The model under review builds one solid part; all positions refer to its coordinate system, in mm. Face numbers are marked on the shaded views. A direction names the side the tool comes from. Coordinates: 2 decimals unless noted, no trailing zeros. Order: outer loops, then holes, each group sorted by start corner. A loop starts at its lowest first (then second) coordinate and runs counter-clockwise, first axis right, second up. Notation, with made-up numbers: (51, -30) -> (60, -30) arc R19 cw to (60, -23) -> close; hole circle Ø1 at (-15.5, 54.25). An arc over 180 degrees is marked (long way). Put each result on its own line as item: value.
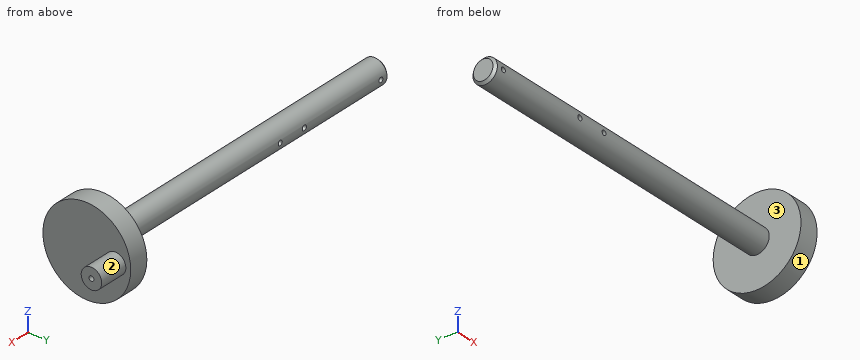
Autodesk Inventor part; units mm, degrees
ref_plane "YZ Plane" through (0, 0, 0) normal (1, 0, 0) x (0, 1, 0)
ref_plane "XZ Plane" through (0, 0, 0) normal (0, 1, 0) x (-1, 0, 0)
ref_plane "XY Plane" through (0, 0, 0) normal (0, 0, 1) x (1, 0, 0)
sketch "Sketch1" plane through (0, 0, 0) normal (0, 0, 1) x (1, 0, 0)
  line L0 (0, 0) -> (72, 0)
  line L1 (68, 2.5) -> (0, 2.5)
  line L2 (0, 2.5) -> (0, 0)
  line L3 (68, 2.5) -> (68, 9)
  line L4 (68, 9) -> (72, 9)
  line L5 (72, 9) -> (72, 0)
revolve "Revolution1" add sketch "Sketch1" angle 360 about axis through (0, 0, 0) along (1, 0, 0)
chamfer "Chamfer1" distance 0.5 angle 45 1 edges at (0, -2.5, 0)
thread "Thread1"
sketch "Sketch2" plane through (72, 0, 0) normal (1, 0, 0) x (0, 0, -1)
  circle A0 centre (0, 5.9) radius 2.1
  circle A1 centre (0, 5.9) radius 0.5
extrude "Extrusion1" add sketch "Sketch2" along normal blind 6
sketch "Sketch3" plane through (0, 0, 0) normal (0, 1, 0) x (-1, 0, 0)
  circle A0 centre (-2, 0) radius 0.5
extrude "Extrusion2" cut sketch "Sketch3" along normal mid plane 10
sketch "Sketch4" plane through (0, 0, 0) normal (0, 1, 0) x (-1, 0, 0)
  circle A0 centre (-27, 0) radius 0.5
extrude "Extrusion3" cut sketch "Sketch4" along normal mid plane 10
sketch "Sketch5" plane through (0, 0, 0) normal (0, 1, 0) x (-1, 0, 0)
  circle A0 centre (-21, 0) radius 0.525
extrude "Extrusion4" cut sketch "Sketch5" along normal mid plane 10
properties part number "shaft"
Item 1: For pin 1 Ø6 at (y, z) = (-2, -0.5) entering from +X; pin 2 Ø2 at (x, y) = (47.5, 5) entering from +Z; pin 3 Ø2 at (x, z) = (11, -0.5) entering from +Y; pin 4 Ø10 at (x, z) = (17.5, -3.5) entering from -Y, all flat-tipped, find the tip position at first contact; note any pin that passes through.
Answers below:
pin 1: x = 72
pin 2: through
pin 3: y = 2.5
pin 4: y = -2.5
Item 2: Consider section B-B on x = 6.5. Write out the cut boundary in (y, z), and give its area (3 significant figures).
Answers below:
outline: circle Ø5 at (0, 0)
area: 19.6 mm^2
Item 3: Consider section D-D on y = -6.5. Write out the cut boundary in (x, z), and give its area (3 significant figures).
Answers below:
outline: (68, -6.22) -> (72, -6.22) -> (72, 6.22) -> (68, 6.22) -> close
area: 49.8 mm^2
Item 4: For the marked faces 1, 2 and 3, list the 3-axis set-ups (+Z, -Z, +X, -X, +Y, -Y) from which the entire face can be reached by the end or side of a thin tool; tool diameter is ignored.
Answers below:
face 1: +X, -X
face 2: +X
face 3: -X
Item 5: Consider section A-A on y = 1.25. Count the separate pieces of the cut face and the enclosed holes in it, and give its area (3 significant figures).
Answers below:
separate pieces: 1
enclosed holes: 3
area: 363 mm^2
Item 6: Consider section C-C on z = 6.75. Write out the cut boundary in (x, y), and give its area (3 significant figures).
Answers below:
outline: (68, -5.95) -> (72, -5.95) -> (72, 5.95) -> (68, 5.95) -> close
area: 47.6 mm^2
Item 7: For line 1 (X direction, y = -1.1, z = 0) (3 decimals); line 2 (Y direction, x = 4.5, z = 0); line 3 (Y direction, x = 42.5, z = -1.5), list the stretches that pass through material, from the lowest coordinate up. Write a range as from..to.
Answers below:
line 1: 0..1.5, 2.5..20.475, 21.525..26.5, 27.5..72
line 2: -2.5..2.5
line 3: -2..2
